from build123d import *

# Parameters (mm, degrees)
F0_R          = 1
F2_DEPTH      = 7
F3_DEPTH      = 10
F3_DEPTH_BACK = 10
F4_W          = 3
F4_H          = 15
F5_DEPTH      = 10
F5_DEPTH_BACK = 10
F6_R          = 0.5
F7_DEPTH      = 25
F8_R          = 4
F8_R_2        = 2.5
F8_R_3        = 1
F9_DEPTH      = 10
F11_DEPTH     = 12
F12_R         = 2.5
F13_DEPTH     = 2
F14_DEPTH     = 25
F15_R         = 5.99999
F16_T1_DEPTH  = 8.00002
F16_T6_ANGLE  = 90
F16_S7_R      = 4
F16_T8_DEPTH  = 7
F16_T12_ANGLE = 90
F16_S13_R     = 4
F16_T14_DEPTH = 7
F16_T18_DEPTH = 19.5703760639
F16_S19_R     = 4
F16_T20_DEPTH = 12
F16_T24_DEPTH = 19.5703760639
F16_S25_R     = 4
F16_T26_DEPTH = 12
F17_R         = 9.99999
F18_R         = 2.5
F18_R_2       = 1
F19_DEPTH     = 1
F20_R         = 2.5


# Not quite as in the source:
# - a fillet or chamfer that OpenCascade refuses, or shapes differently, is made with other operations: its cross-section is extruded or revolved along the edge and cut away or added
# - a fillet or chamfer is up to 0.001 mm smaller than in the source, because OpenCascade refuses the exact size


with BuildPart() as f2:
    # F0 (on Right) → F2 (new body)
    with BuildSketch(Plane.YZ):
        with BuildLine():
            ThreePointArc((-2.5, 4.8733971724), (-3.0435645354, 5.7631536934), (-4.0833333333, 5.6856300345))
            ThreePointArc((-4.0833333333, 5.6856300345), (-7, 0), (-4.0833333333, -5.6856300345))
            ThreePointArc((-4.0833333333, -5.6856300345), (-3.0435645354, -5.7631536934), (-2.5, -4.8733971724))
            Line((-2.5, -4.8733971724), (-2.5, 0))
            Line((-2.5, 0), (-2.5, 4.8733971724))
        make_face()
        with Locations((-5, 0)):
            Circle(F0_R, mode=Mode.SUBTRACT)
    extrude(amount=-F2_DEPTH)



with BuildPart() as f2b:
    # F0 (on Right) → F2, piece 2 (new body)
    with BuildSketch(Plane.YZ):
        with BuildLine():
            Line((2.5, 4.8733971724), (2.5, 0))
            Line((2.5, 0), (2.5, -4.8733971724))
            ThreePointArc((2.5, -4.8733971724), (3.0435645354, -5.7631536934), (4.0833333333, -5.6856300345))
            ThreePointArc((4.0833333333, -5.6856300345), (7, 0), (4.0833333333, 5.6856300345))
            ThreePointArc((4.0833333333, 5.6856300345), (3.0435645354, 5.7631536934), (2.5, 4.8733971724))
        make_face()
        with Locations((5, 0)):
            Circle(F0_R, mode=Mode.SUBTRACT)
    extrude(amount=-F2_DEPTH)


with BuildPart() as f2_1:
    add(f2.part)

    add(f2b.part)  # F3 merges F2b
    # F1 (on Front) → F3 (join, two sides)
    with BuildSketch(Plane.XZ) as f3_sk:
        Polygon((0, -12), (-7, -12), (-7, 10), (-10, 10), (-10, -27), (0, -27), align=None)
    extrude(amount=F3_DEPTH)
    extrude(f3_sk.sketch, amount=-F3_DEPTH_BACK)

    # F4 (on Front) → F5 (cut, two sides)
    with BuildSketch(Plane.XZ) as f5_sk:
        with Locations((-1.5, 0)):
            Rectangle(F4_W, F4_H)
    extrude(amount=-F5_DEPTH, mode=Mode.SUBTRACT)
    extrude(f5_sk.sketch, amount=F5_DEPTH_BACK, mode=Mode.SUBTRACT)

    # F6
    f6_edges = [f2_1.edges().sort_by_distance(p)[0] for p in [
        (-3, -7, 0),
        (-3, 2.5, 0),
        (-3, -3.043565, 5.763154),
        (-3, -3.043565, -5.763154),
        (-3, -2.5, 0),
        (-3, 7, 0),
        (-3, 3.043565, -5.763154),
        (-3, 3.043565, 5.763154),
    ]]
    fillet(f6_edges, radius=F6_R)

    # F0 (on Right) → F7 (cut)
    with BuildSketch(Plane.YZ):
        with Locations((-8, -18)):
            Circle(F0_R)
        with Locations((8, -18)):
            Circle(F0_R)
    extrude(amount=-F7_DEPTH, mode=Mode.SUBTRACT)

    # F8 (on Right) → F9 (join)
    with BuildSketch(Plane.YZ):
        with Locations((8, -18)):
            Circle(F8_R)
        with Locations((8, -18)):
            Circle(F8_R_2, mode=Mode.SUBTRACT)
        with Locations((-8, -18)):
            Circle(F8_R)
        with Locations((-8, -18)):
            Circle(F8_R_2, mode=Mode.SUBTRACT)
        with Locations((8, -18)):
            Circle(F8_R_2)
        with Locations((8, -18)):
            Circle(F8_R_3, mode=Mode.SUBTRACT)
        with Locations((-8, -18)):
            Circle(F8_R_2)
        with Locations((-8, -18)):
            Circle(F8_R_3, mode=Mode.SUBTRACT)
    extrude(amount=-F9_DEPTH)

    # F10 (on face) → F11 (cut)
    with BuildSketch(Plane(origin=(0, 0, -27), x_dir=(1, 0, 0), z_dir=(0, 0, -1))):
        with BuildLine():
            Line((0, -5), (0, 5))
            ThreePointArc((0, 5), (-5, 0), (0, -5))
        make_face()
    extrude(amount=-F11_DEPTH, mode=Mode.SUBTRACT)

    # F12 (on face) → F13 (cut)
    with BuildSketch(Plane(origin=(-10, 0, 0), x_dir=(0, -1, 0), z_dir=(-1, 0, 0))):
        with Locations((-8, -18)):
            Circle(F12_R)
        with Locations((8, -18)):
            Circle(F12_R)
    extrude(amount=-F13_DEPTH, mode=Mode.SUBTRACT)

    # F0 (on Right) → F14 (cut)
    with BuildSketch(Plane.YZ):
        with Locations((-5, 0)):
            Circle(F0_R)
        with Locations((5, 0)):
            Circle(F0_R)
    extrude(amount=-F14_DEPTH, mode=Mode.SUBTRACT)

    # F15 (radius 6 in the source; OpenCascade refuses exactly that, so slightly less here)
    f15_edges = [f2_1.edges().sort_by_distance(p)[0] for p in [
        (-10, 10, -24.232051),
        (-10, -10, -24.232051),
    ]]
    fillet(f15_edges, radius=F15_R)

    # F16: chamfer of 2 x 6 on 5 edges, made by hand

    # F16_s2 → F16_t1 (cut)
    with BuildSketch(Plane.XZ.offset(-4.00001)):
        Polygon((-10, -21), (-8, -27), (-10, -27), align=None)
    extrude(amount=F16_T1_DEPTH, mode=Mode.SUBTRACT)


with BuildPart() as f16_tool4:
    # F16_s5 → F16_t6 (revolve)
    with BuildSketch(Plane.XZ.offset(-4.00001)):
        Polygon((-8, -27), (-10, -21), (-10, -27), align=None)
    revolve(axis=Axis((-4.00001, 4.00001, -27), (0, 0, -1)), revolution_arc=F16_T6_ANGLE)

    # F16_s7 → F16_t8 (cut, symmetric)
    with BuildSketch(Plane.YZ.offset(-7)):
        with Locations((8, -18)):
            Circle(F16_S7_R)
    extrude(amount=F16_T8_DEPTH, both=True, mode=Mode.SUBTRACT)


with BuildPart() as f2_2:
    add(f2_1.part)

    # F16_t3: cut F16_tool4
    add(f16_tool4.part, mode=Mode.SUBTRACT)


with BuildPart() as f16_tool10:
    # F16_s11 → F16_t12 (revolve)
    with BuildSketch(Plane.XZ.offset(4.00001)):
        Polygon((-8, -27), (-10, -21), (-10, -27), align=None)
    revolve(axis=Axis((-4.00001, -4.00001, -27), (0, 0, 1)), revolution_arc=F16_T12_ANGLE)

    # F16_s13 → F16_t14 (cut, symmetric)
    with BuildSketch(Plane.YZ.offset(-7)):
        with Locations((-8, -18)):
            Circle(F16_S13_R)
    extrude(amount=F16_T14_DEPTH, both=True, mode=Mode.SUBTRACT)


with BuildPart() as f2_3:
    add(f2_2.part)

    # F16_t9: cut F16_tool10
    add(f16_tool10.part, mode=Mode.SUBTRACT)


with BuildPart() as f16_tool16:
    # F16_s17 → F16_t18 (new body)
    with BuildSketch(Plane.YZ.offset(-4.00001)):
        Polygon((-8, -27), (-10, -21), (-10, -27), align=None)
    extrude(amount=F16_T18_DEPTH)

    # F16_s19 → F16_t20 (cut, symmetric)
    with BuildSketch(Plane.YZ.offset(5.8)):
        with Locations((-8, -18)):
            Circle(F16_S19_R)
    extrude(amount=F16_T20_DEPTH, both=True, mode=Mode.SUBTRACT)


with BuildPart() as f2_4:
    add(f2_3.part)

    # F16_t15: cut F16_tool16
    add(f16_tool16.part, mode=Mode.SUBTRACT)


with BuildPart() as f16_tool22:
    # F16_s23 → F16_t24 (new body)
    with BuildSketch(Plane.YZ.offset(-4.00001)):
        Polygon((8, -27), (10, -21), (10, -27), align=None)
    extrude(amount=F16_T24_DEPTH)

    # F16_s25 → F16_t26 (cut, symmetric)
    with BuildSketch(Plane.YZ.offset(5.8)):
        with Locations((8, -18)):
            Circle(F16_S25_R)
    extrude(amount=F16_T26_DEPTH, both=True, mode=Mode.SUBTRACT)


with BuildPart() as f2_5:
    add(f2_4.part)

    # F16_t21: cut F16_tool22
    add(f16_tool22.part, mode=Mode.SUBTRACT)

    # F17 (radius 10 in the source; OpenCascade refuses exactly that, so slightly less here)
    f17_edges = [f2_5.edges().sort_by_distance(p)[0] for p in [
        (-8.5, -10, 10),
        (-8.5, 10, 10),
    ]]
    fillet(f17_edges, radius=F17_R)

    # F18 (on face) → F19 (cut)
    with BuildSketch(Plane(origin=(-10, 0, 0), x_dir=(0, -1, 0), z_dir=(-1, 0, 0))):
        with Locations((-5, 0)):
            Circle(F18_R)
        with Locations((-5, 0)):
            Circle(F18_R_2, mode=Mode.SUBTRACT)
        with Locations((5, 0)):
            Circle(F18_R)
        with Locations((5, 0)):
            Circle(F18_R_2, mode=Mode.SUBTRACT)
    extrude(amount=-F19_DEPTH, mode=Mode.SUBTRACT)

    # F20
    f20_edges = [f2_5.edges().sort_by_distance(p)[0] for p in [
        (-3.5, 10, -12),
        (-3.5, -10, -12),
    ]]
    fillet(f20_edges, radius=F20_R)


solid = f2_5.part
Verification items for the finished model (mm, model axes). A direction names the side the tool comes from. Round coordinates to 2 decimals unless told otherwise and drop trailing zeros. Loops run counter-clockwise (first coordinate to the right, second up) from the corner with the lowest first, then second, coordinate; pieces in that order, holes last. Notation, with made-up numbers: (-35.75, 62.25) - (16.25, 62.25) arc R16 ccw to (16.25, 66.25) - close; hole circle Ø3 at (-34, 89.25). An arc over 180 degrees is marked (long way). Use a Markdown table: item, result. Add a question column.
1. Section check A-A, the plane x = -0.75. Give the number of separate pieces and of enclosed holes in the cut face, plus the area to 3 significant figures.
2. Release check for a two-part mould opening along Z. For faces 4 (the face through (-2, -9, -24)), 5 (the face through (-5, 7, 0)), 6 (the face through (-5, 0, -21)), 7 (the face through (-9, 10.5, -17.9)) record: released by +Z, released by -Z, zero draft, split by the parting line, or undercut.
3. Access from +Z, -Z, +X, -X, +Y, -Y to the whole of each face (thin tool, end or side, straight path). Record for faces 1 (the face through (-3, 3.6, -0.1)), 2 (the face through (-7, 0, -2)), 3 (the face through (-8, -9, -19)).
4. Gauge pin test, flat ends, axial feed: pin 1 (1 mm diameter, centred on x = -2, z = -14.5, fed in from -Y); pin 2 (4 mm diameter, centred on y = 8, z = -18, fed in from -X); pin 3 (3 mm diameter, centred on x = -6.5, z = -11.5, fed in from -Y). Record the tip position at first contact, or that the pin passes through.
5. Section check B-B, the plane z = -17.5. Record the boundary of the cut face in (x, y).
6. Thickness scan on probe 1 along Z at (x, y) = (-4.85, 5); probe 2 along X at (y, z) = (-8.5, -16.5); probe 3 along X at (y, z) = (2.25, -6). Record the ranges inside material, lowest first. Write a range as [from, to].
7. Section check C-C, the plane z = -23. Record the boundary of the cut face in (x, y).
8. Section check D-D, the plane z = -11. Record the boundary of the cut face in (x, y), plus the area to 3 significant figures.
Checks:
| question | item | result |
|---|---|---|
| 1 | separate pieces | 1 |
| 1 | enclosed holes | 2 |
| 1 | area | 180 mm^2 |
| 2 | face 4 | released by -Z |
| 2 | face 5 | undercut |
| 2 | face 6 | zero draft |
| 2 | face 7 | undercut |
| 3 | face 1 | +Z, +X, +Y, -Y |
| 3 | face 2 | +X |
| 3 | face 3 | -X |
| 4 | pin 1 | stops at y = -10.65 |
| 4 | pin 2 | stops at x = -8 |
| 4 | pin 3 | stops at y = -10 |
| 5 | outline | (-10, -11.97) - (0, -11.97) - (0, -8.87) - (-8, -8.87) - (-8, -10.45) - (-10, -10.45) - close; (-10, -5.55) - (-8, -5.55) - (-8, -7.13) - (0, -7.13) - (0, -5) arc R5 cw to (0, 5) - (0, 7.13) - (-8, 7.13) - (-8, 5.55) - (-10, 5.55) - close; (-10, 10.45) - (-8, 10.45) - (-8, 8.87) - (0, 8.87) - (0, 11.97) - (-10, 11.97) - close |
| 6 | probe 1 | z = [-27, -12], [-4.9, -1], [1, 4.9] |
| 6 | probe 2 | x = [-8, 0] |
| 6 | probe 3 | x = [-10, -7] |
| 7 | outline | (-9.33, -4) arc R5.33 ccw to (-4, -9.33) - (0, -9.33) - (0, -5) arc R5 cw to (0, 5) - (0, 9.33) - (-4, 9.33) arc R5.33 ccw to (-9.33, 4) - close |
| 8 | outline | (-10, -10) - (-7, -10) - (-7, 10) - (-10, 10) - close |
| 8 | area | 60.0 mm^2 |
